For this review, take the finished solid that the model builds, in its own axes (mm). Face numbers are marked on the shaded views. A direction names the side the tool comes from. Give positions to 0.01 mm unless a question says otherwise; leave off trailing zeros. Order: outer loops, then holes, each group sorted by start corner. A loop starts at its lowest first (then second) coordinate and runs counter-clockwise, first axis right, second up.
Item 1: Consider section B-B (y = -2.75). Give the boundary of the cut face in (x, z), plus the area to 3 significant figures.
Item 2: Consider section C-C (z = 20.5). Give the boundary of the cut face in (x, y).
Item 3: For probe 1 along X at (y, z) = (1.25, 13.5); probe 2 along Y at (x, z) = (2.75, 17); probe 3 along X at (y, z) = (-4.5, 12), list the stretches that pass through material, from the lowest coordinate up.
Item 4: Machinability: for the marked faces 4, 5 and 6, which of the approach directions +Z, -Z, +X, -X, +Y, -Y give a long, thin tool a straight path to every point of the face, cutting with its end or side? Answer none if there is none.
Item 5: Consider section D-D (x = -16.75). Give the boundary of the cut face in (y, z), plus the area to 3 significant figures.
Item 6: For P1, Ø3, axis at y = -1, z = 12, coming from the -X side; P2, Ø3, axis at x = -7, y = -4, coming from the +Z side, all flat-tipped, find the tip position at first contact; note any pin that passes through.
Item 7: The part is to be moulded in two halves that separate along Z. For the marked faces 1, 2 and 3, say which applies: released by +Z, released by -Z, zero draft, split by the parting line, or undercut.
Item 8: Consider section A-A (z = 13.5). Give the boundary of the cut face in (x, y), plus the area to 3 significant figures.
```python
from build123d import *

# Parameters (mm, degrees)
SKETCH1_W           = 10.758936
SKETCH1_H           = 10.375
SKETCH1_W_2         = 6.758936
SKETCH1_H_2         = 6.375
BOSS_EXTRUDE1_DEPTH = 18
BOSS_EXTRUDE2_DEPTH = 2
BOSS_EXTRUDE3_REACH = 21.49
SKETCH3_W           = 10.758936
SKETCH3_H           = 10.375
SKETCH3_W_2         = 6.758936
SKETCH3_H_2         = 6.375
BOSS_EXTRUDE7_DEPTH = 10.375
BOSS_EXTRUDE8_DEPTH = 10.375


with BuildPart() as part:
    # Sketch1 → Boss-Extrude1 (new body)
    with BuildSketch(Plane.XY):
        Rectangle(SKETCH1_W, SKETCH1_H)
        Rectangle(SKETCH1_W_2, SKETCH1_H_2, mode=Mode.SUBTRACT)
    extrude(amount=BOSS_EXTRUDE1_DEPTH)

    # Sketch2 → Boss-Extrude2 (add)
    with BuildSketch(Plane(origin=(0, -3.1875, 0), x_dir=(1, 0, 0), z_dir=(0, 1, 0))):
        Polygon((3.379468, -18), (-3.550178456, -24.929646456), (-3.379468, -18), align=None)
    extrude(amount=-BOSS_EXTRUDE2_DEPTH)

    # Boss-Extrude3: up to this face of the body (flat: up to its plane)
    boss_extrude3_end = Plane(part.part.faces().sort_by_distance((-0.085355228, -4.1875, 21.464823228))[0])
    # Sketch3 → Boss-Extrude3 (add, up to the picked face)
    with BuildSketch(Plane.XY.offset(18), mode=Mode.PRIVATE) as boss_extrude3_sk1:
        Rectangle(SKETCH3_W, SKETCH3_H)
        Rectangle(SKETCH3_W_2, SKETCH3_H_2, mode=Mode.SUBTRACT)
    boss_extrude3_tool1 = split(extrude(boss_extrude3_sk1.sketch, amount=BOSS_EXTRUDE3_REACH, mode=Mode.PRIVATE), bisect_by=boss_extrude3_end, keep=Keep.BOTH, mode=Mode.PRIVATE)
    add(boss_extrude3_tool1.solids().sort_by(Axis((0, -5.038036, 18), (0, 0, 1)))[0])

    # Sketch7 → Boss-Extrude7 (add)
    with BuildSketch(Plane(origin=(0, -5.1875, 0), x_dir=(-1, 0, 0), z_dir=(0, -1, 0))):
        Polygon((5.379468, -26.758936), (19.868355394, -30.641221677), (19.868355394, -22.641221677), (5.379468, -18.758936), align=None)
    extrude(amount=-BOSS_EXTRUDE7_DEPTH)

    # Sketch8 → Boss-Extrude8 (add)
    with BuildSketch(Plane(origin=(0, -5.1875, 0), x_dir=(-1, 0, 0), z_dir=(0, -1, 0))):
        Polygon((5.379468, -26.758936), (-5.379468, -18), (-3.379468, -18), align=None)
    extrude(amount=-BOSS_EXTRUDE8_DEPTH)


solid = part.part
```
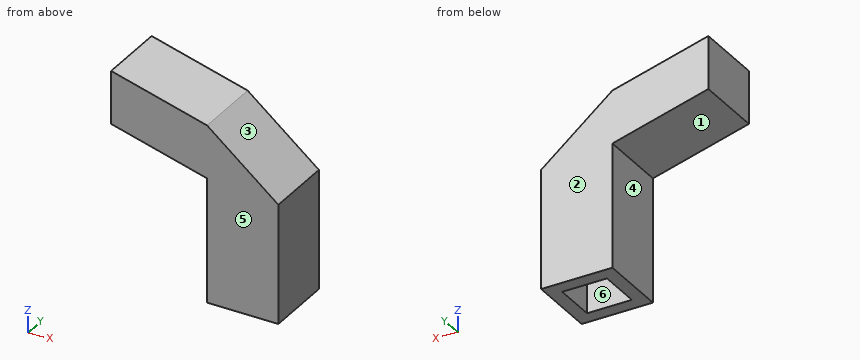
Resolved:
1. outline: (-19.87, 22.64) - (-5.38, 18.76) - (-5.38, 0) - (-3.38, 0) - (-3.38, 24.76) - (3.38, 18) - (3.38, 0) - (5.38, 0) - (5.38, 18) - (-5.38, 26.76) - (-19.87, 30.64) - close
1. area: 212 mm2
2. outline: (-11.88, -5.19) - (2.31, -5.19) - (2.31, 5.19) - (-11.88, 5.19) - close; hole (-3.38, -3.19) - (0.88, -3.19) - (0.88, 3.19) - (-3.38, 3.19) - close
3. probe 1: x = -5.38 to -3.38, 3.38 to 5.38
3. probe 2: y = -5.19 to -3.19, 3.19 to 5.19
3. probe 3: x = -5.38 to 5.38
4. face 4: -Z, -X, +Y, -Y
4. face 5: +Z, -Z, +X, -X, -Y
4. face 6: -Z
5. outline: (-5.19, 21.81) - (5.19, 21.81) - (5.19, 29.81) - (-5.19, 29.81) - close
5. area: 83.0 mm2
6. P1: stops at x = -5.38
6. P2: stops at z = 27.6
7. face 1: released by -Z
7. face 2: zero draft
7. face 3: released by +Z
8. outline: (-5.38, -5.19) - (5.38, -5.19) - (5.38, 5.19) - (-5.38, 5.19) - close; hole (-3.38, -3.19) - (3.38, -3.19) - (3.38, 3.19) - (-3.38, 3.19) - close
8. area: 68.5 mm2
